```python
from build123d import *

# Parameters (mm, degrees)
SKETCH1_W           = 63.5
SKETCH1_H           = 20.32
BOSS_EXTRUDE1_DEPTH = 20.32
CUT_EXTRUDE2_DEPTH  = 20.32
FILLET1_R           = 2.54
SKETCH3_R           = 2.54
BOSS_EXTRUDE2_DEPTH = 15.24
FILLET2_R           = 2.54
CUT_EXTRUDE3_START  = -5.08
SKETCH4_R           = 2.54
CUT_EXTRUDE3_DEPTH  = 5.08


with BuildPart() as part:
    # Sketch1 → Boss-Extrude1 (new body)
    with BuildSketch(Plane.XY):
        Rectangle(SKETCH1_W, SKETCH1_H)
    extrude(amount=BOSS_EXTRUDE1_DEPTH)

    # Sketch2 → Cut-Extrude2 (cut)
    with BuildSketch(Plane(origin=(31.75, 0, 0), x_dir=(0, 0, -1), z_dir=(1, 0, 0))):
        with BuildLine():
            Line((-20.32, 2.54), (-20.32, 10.16))
            Line((-20.32, 10.16), (-12.7, 10.16))
            ThreePointArc((-12.7, 10.16), (-18.088153673, 7.928153673), (-20.32, 2.54))
        make_face()
        with BuildLine():
            Line((-7.62, 10.16), (0, 10.16))
            Line((0, 10.16), (0, 2.54))
            ThreePointArc((0, 2.54), (-2.231846327, 7.928153673), (-7.62, 10.16))
        make_face()
        with BuildLine():
            Line((-7.62, -10.16), (0, -10.16))
            Line((0, -10.16), (0, -2.54))
            ThreePointArc((0, -2.54), (-2.231846327, -7.928153673), (-7.62, -10.16))
        make_face()
        with BuildLine():
            Line((-12.7, -10.16), (-20.32, -10.16))
            Line((-20.32, -10.16), (-20.32, -2.54))
            ThreePointArc((-20.32, -2.54), (-18.088153673, -7.928153673), (-12.7, -10.16))
        make_face()
    extrude(amount=-CUT_EXTRUDE2_DEPTH, mode=Mode.SUBTRACT)

    # Fillet1
    fillet1_edges = [part.edges().sort_by_distance(p)[0] for p in [
        (31.75, 0, 0),
        (31.75, 0, 20.32),
        (31.75, -10.16, 10.16),
        (31.75, 10.16, 10.16),
        (31.75, -7.928153673, 18.088153673),
        (31.75, -7.928153673, 2.231846327),
        (31.75, 7.928153673, 2.231846327),
        (31.75, 7.928153673, 18.088153673),
    ]]
    fillet(fillet1_edges, radius=FILLET1_R)

    # Sketch3 → Boss-Extrude2 (add)
    with BuildSketch(Plane(origin=(0, 10.16, 0), x_dir=(1, 0, 0), z_dir=(0, 1, 0))):
        with Locations(Location((20.4017153, -10.16, 0), (0, 0, 270))):
            Circle(SKETCH3_R)
    extrude(amount=BOSS_EXTRUDE2_DEPTH)

    # Fillet2
    fillet2_edges = [part.edges().sort_by_distance(p)[0] for p in [
        (-31.75, 0, 20.32),
        (-31.75, 0, 0),
        (-31.75, -10.16, 10.16),
        (-31.75, 10.16, 10.16),
    ]]
    fillet(fillet2_edges, radius=FILLET2_R)

    # Sketch4 → Cut-Extrude3 (cut)
    with BuildSketch(Plane(origin=(0, 25.4, 0), x_dir=(1, 0, 0), z_dir=(0, 1, 0)).offset(CUT_EXTRUDE3_START)):
        with Locations(Location((20.4017153, -10.16, 0), (0, 0, 270))):
            Circle(SKETCH4_R)
    extrude(amount=CUT_EXTRUDE3_DEPTH, mode=Mode.SUBTRACT)


solid = part.part
```
Geometry: final body of the model. Coordinates: model frame, mm. A direction names the side the tool comes from. Round coordinates to 2 decimals unless told otherwise and drop trailing zeros. Order: outer loops, then holes, each group sorted by start corner. A loop starts at its lowest first (then second) coordinate and runs counter-clockwise, first axis right, second up. Notation, with made-up numbers: (-40, 33.25) - (11, 33.25) arc R33 ccw to (11, 70.25) - close; hole circle Ø9 at (64, -31.75). An arc over 180 degrees is marked (long way). Write item = value, one per line. Start each with the question number.
Q1. Cut plane A-A on z = 10.16. Return the cut outline in (x, y), and give its area (3 significant figures).
Q2. Cut plane B-B on x = 27. Return the cut outline in (y, z).
Q3. Cut plane C-C on x = 0. Return the cut outline in (y, z), and give its area (3 significant figures).
Q4. Pin query (flat end, axial travel): pin 1 (3 mm diameter, centred on x = -4, z = 14, fed in from +Y); pin 2 (3 mm diameter, centred on x = 7, y = 13.5, fed in from -Z). Return the tip coordinate at first contact, or that it passes through.
Q5. Access query for faces 1 (the cylindrical face through (20.444, 7.869, 2.173)), 2 (the cylindrical face through (20.444, -7.869, 2.173)), 3 (the cylindrical face through (20.444, 7.987, 18.029)). Directions: +Z, -Z, +X, -X, +Y, -Y. A direction counts if a zero-diameter tool reaches every point of the face in a straight line with its end or side. Return the directions, or none.
Q6. Ray query, line 1 (Y direction, x = -13.5, z = 5); line 2 (Z direction, x = 28, y = -3.5); line 3 (Y direction, x = 21.5, z = 3). Return the intervals inside material, ascending. Write a range as from..to.
Outcome:
q1.outline = (-31.75, -7.62) arc R2.54 ccw to (-29.21, -10.16) - (29.21, -10.16) arc R2.54 ccw to (31.75, -7.62) - (31.75, 7.62) arc R2.54 ccw to (29.21, 10.16) - (22.94, 10.16) - (22.94, 20.32) - (17.86, 20.32) - (17.86, 10.16) - (-29.21, 10.16) arc R2.54 ccw to (-31.75, 7.62) - close
q1.area = 1,340 mm^2
q2.outline = (-10.16, 7.62) arc R7.62 ccw to (-2.54, 0) - (2.54, 0) arc R7.62 ccw to (10.16, 7.62) - (10.16, 12.7) arc R7.62 ccw to (2.54, 20.32) - (-2.54, 20.32) arc R7.62 ccw to (-10.16, 12.7) - close
q3.outline = (-10.16, 0) - (10.16, 0) - (10.16, 20.32) - (-10.16, 20.32) - close
q3.area = 413 mm^2
q4.pin_1 = 10.16
q4.pin_2 = through
q5.face_1 = -Z, +X, +Y
q5.face_2 = -Z, +X, -Y
q5.face_3 = +Z, +X, +Y
q6.line_1 = -10.16..10.16
q6.line_2 = 0.06..20.26
q6.line_3 = -8.6..8.6
